Build history of the part. All positions in model axes, mm. Face numbers are marked on the shaded views. Round coordinates to 2 decimals unless told otherwise and drop trailing zeros. Write each loop counter-clockwise with the first axis right and the second up, starting at its lowest first coordinate (ties: lowest second). Pieces come first, ordered by that corner, then holes.
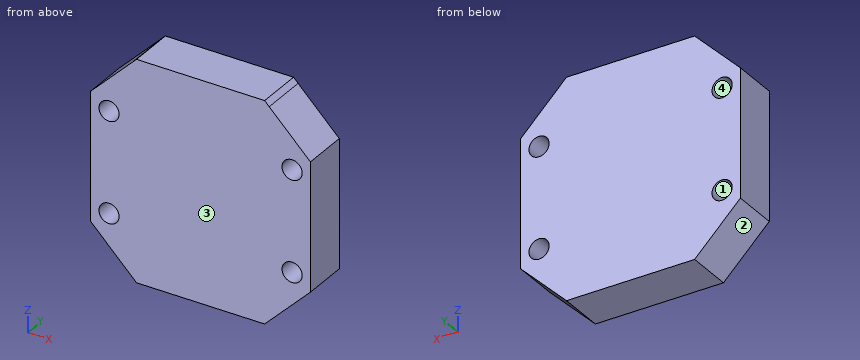
Autodesk Inventor part; units mm, degrees
ref_plane "YZ Plane" through (0, 0, 0) normal (1, 0, 0) x (0, 1, 0)
ref_plane "XZ Plane" through (0, 0, 0) normal (0, 1, 0) x (-1, 0, 0)
ref_plane "XY Plane" through (0, 0, 0) normal (0, 0, 1) x (1, 0, 0)
sketch "Sketch1" plane through (0, 0, 0) normal (0, 1, 0) x (-1, 0, 0)
  line L0 (10.5005, 23.9999) -> (3.4998, 23.9999)
  line L1 (3.4998, 23.9999) -> (10.5005, 23.9999)
  line L2 (-4.9999, 18.9997) -> (-4.9999, 5.0001)
  line L3 (-0.5002, 23.5006) -> (-4.9999, 18.9997)
  line L4 (-4.9999, 18.9997) -> (-4.9999, 5.0001)
  line L5 (0.0015, 0) -> (13.9982, -0.0002)
  line L6 (-4.9999, 5.0001) -> (0.0015, 0)
  line L7 (0.0015, 0) -> (13.9982, -0.0002)
  line L8 (13.9982, -0.0002) -> (18.9999, 5.0029)
  line L9 (18.9999, 5.0029) -> (19.0001, 19)
  line L10 (18.9999, 5.0029) -> (19.0001, 19)
  line L11 (19.0001, 19) -> (14.4994, 23.4994)
  circle A0 centre (17, 17.4999) radius 0.8
  circle A1 centre (17, 17.4999) radius 0.8
  circle A2 centre (17, 6.5) radius 0.8
  circle A3 centre (17, 6.5) radius 0.8
  circle A4 centre (-3, 17.5) radius 0.8
  circle A5 centre (-3, 17.5) radius 0.8
  circle A6 centre (-3, 6.5) radius 0.8
  circle A7 centre (-3, 17.5) radius 0.8
  line L12 (19.0001, 19) -> (19.0001, 16.4173)
  line L13 (19.0001, 19) -> (19, 15.3998)
  line L14 (19.0001, 19) -> (19, 15.3998)
  line L15 (19.0001, 19) -> (18.3991, 19.6008)
  line L16 (19.0001, 19) -> (18.3998, 19.6001)
  line L17 (19.0001, 19) -> (19, 11.9999)
  line L18 (19, 11.9999) -> (-4.9999, 11.9999)
  line L19 (19, 11.9999) -> (7, 11.9999)
  line L20 (6.9998, -0.0001) -> (7.0002, 23.9999)
  line L21 (-4.8205, 19.6001) -> (-4.8205, 19.6005)
  line L22 (-2.9994, 19.6006) -> (-2.9994, 19.6001)
  line L23 (10.5005, 23.9999) -> (13.9988, 23.9999)
  line L24 (14.4994, 23.4994) -> (13.9988, 23.9999)
  line L25 (3.4998, 23.9999) -> (-0.001, 23.9999)
  line L26 (-0.5002, 23.5006) -> (-0.001, 23.9999)
  point P0 (0, 0)
  point P1 (0, 0)
  point P2 (10, 14.9997)
  point P3 (4.0003, 14.9997)
  point P4 (4.0003, 8.0001)
  point P5 (7, 14.9997)
  point P6 (7, 14.9997)
  point P7 (7, 14.9997)
  point P8 (7, 11.9999)
  point P9 (-4.9999, 15.4002)
  point P10 (-4.9999, 8.6003)
  point P11 (-4.3996, 4.4)
  point P12 (18.3968, 4.3997)
  point P13 (18.9999, 8.6)
  point P14 (19, 15.3998)
  point P15 (18.9999, 8.6)
  dimension "d2" = 1.6
extrude "Extrusion1" add sketch "Sketch1" along normal blind 5
hole "Hole1" at (-17, 0, 6.5) at (-17, 0, 17.4999) at (3, 0, 17.5) at (3, 0, 6.5) direction (0, 1, 0) diameter 2.2 end through all
properties part number "marcor_isolator"
1) Mould opens along X. For the marked faces 1, 2, 3 and 4 say: released by +X, released by -X, zero draft, split by the parting line, or undercut.
Results:
face 1: undercut
face 2: released by -X
face 3: zero draft
face 4: undercut
2) Wall check: L1, parallel to X at y = 1.2, z = 17.5; L2, parallel to Z at x = 2, y = 2.25; L3, parallel to Z at x = 3, y = 2.8. Give the ranges that are in metal, low to high.
Results:
L1: x = -19 to -18.1, -15.9 to 1.9, 4.1 to 5
L2: z = 2 to 6.04, 6.96 to 17.04, 17.96 to 22
L3: z = 3 to 5.4, 7.6 to 16.4, 18.6 to 21
3) Slice it at B-B (x = -16.25). Write the cut outline in (y, z), plus the area to 3 significant figures.
Results:
outline: (0, 2.25) - (5, 2.25) - (5, 5.7) - (0, 5.7) - close; (0, 7.3) - (5, 7.3) - (5, 16.7) - (0, 16.7) - close; (0, 18.3) - (5, 18.3) - (5, 21.75) - (0, 21.75) - close
area: 81.4 mm2
4) Slice it at C-C (z = 17.5). Write the cut outline in (x, y), plus the area to 3 significant figures.
Results:
outline: (-19, 0) - (-18.1, 0) - (-18.1, 5) - (-19, 5) - close; (-15.9, 0) - (1.9, 0) - (1.9, 5) - (-15.9, 5) - close; (4.1, 0) - (5, 0) - (5, 5) - (4.1, 5) - close
area: 98.0 mm2
5) Pin check, flat tips, straight feed: pin 1 Ø1 at (x, y) = (-15.5, 1.5) entering from +Z; pin 2 Ø2 at (x, z) = (3, 6.5) entering from +Y; pin 3 Ø1 at (x, y) = (-16, 1) entering from -Z. Stop position of each tip, or through.
Results:
pin 1: stops at z = 23
pin 2: passes through
pin 3: stops at z = 1.5
6) Slice it at A-A (y = 1.35). Write the cut outline in (x, z).
Results:
outline: (-19, 5) - (-14, 0) - (0, 0) - (5, 5) - (5, 19) - (0.5, 23.5) - (0, 24) - (-14, 24) - (-14.5, 23.5) - (-19, 19) - close; hole circle Ø2.2 at (-17, 6.5); hole circle Ø2.2 at (-17, 17.5); hole circle Ø2.2 at (3, 6.5); hole circle Ø2.2 at (3, 17.5)
7) Slice it at D-D (z = 20.75). Write the cut outline in (x, y).
Results:
outline: (-17.25, 0) - (3.25, 0) - (3.25, 5) - (-17.25, 5) - close
